For this review, use the dimensioned drawing (mm, ordinates from the lowest corner) and the shaded views. A direction names the side the tool comes from. Coordinates: 2 decimals unless noted, no trailing zeros. Order: outer loops, then holes, each group sorted by start corner. A loop starts at its lowest first (then second) coordinate and runs counter-clockwise, first axis right, second up. Notation, with made-up numbers: (67.5, -33.75) -> (122.5, -33.75) arc R36 cw to (122.5, 1.25) -> close; hole circle Ø10 at (-10, 76). An arc over 180 degrees is marked (long way). Use one line per item in the form item = value. Start each with the question number.
(1) Mouldability with a two-part tool opening along X and no side actions: class the marked faces 3, 4 and 5 as +X half, -X half, draft (parallel to the pull), parting line (faces both ways), or undercut.
(2) Take a section at C-C (y = 19). State the section outline as (x, z) points.
(3) Take a section at D-D (y = 8). State the section outline as (x, z) points, then the cut area to 3 significant figures.
(4) Take a section at A-A (x = 17.5). State the section outline as (y, z) points, then the cut area to 3 significant figures.
(5) Take a section at B-B (z = 17.5). State the section outline as (x, y) points.
(6) Wall thickness on line 1 along X through (y, z) = (20.5, 17.5); line 2 along Z through (x, y) = (17.5, 10.5): over which ranges is each line inside the solid? List them lowest first.
(7) Insertion check: pin 1 Ø4 at (y, z) = (22.5, 20) entering from +X; pin 2 Ø2 at (x, y) = (17.5, 15) entering from +Z; pin 3 Ø5 at (y, z) = (13.5, 7.5) entering from +X. Each pin has a flat end and moves straight along its axis. Give the tip position at first contact, or say it passes through.
(8) For the marked faces 1 and 2, list the 3-axis set-ups (+Z, -Z, +X, -X, +Y, -Y) from which the entire face can be reached by the end or side of a thin tool; tool diameter is ignored.
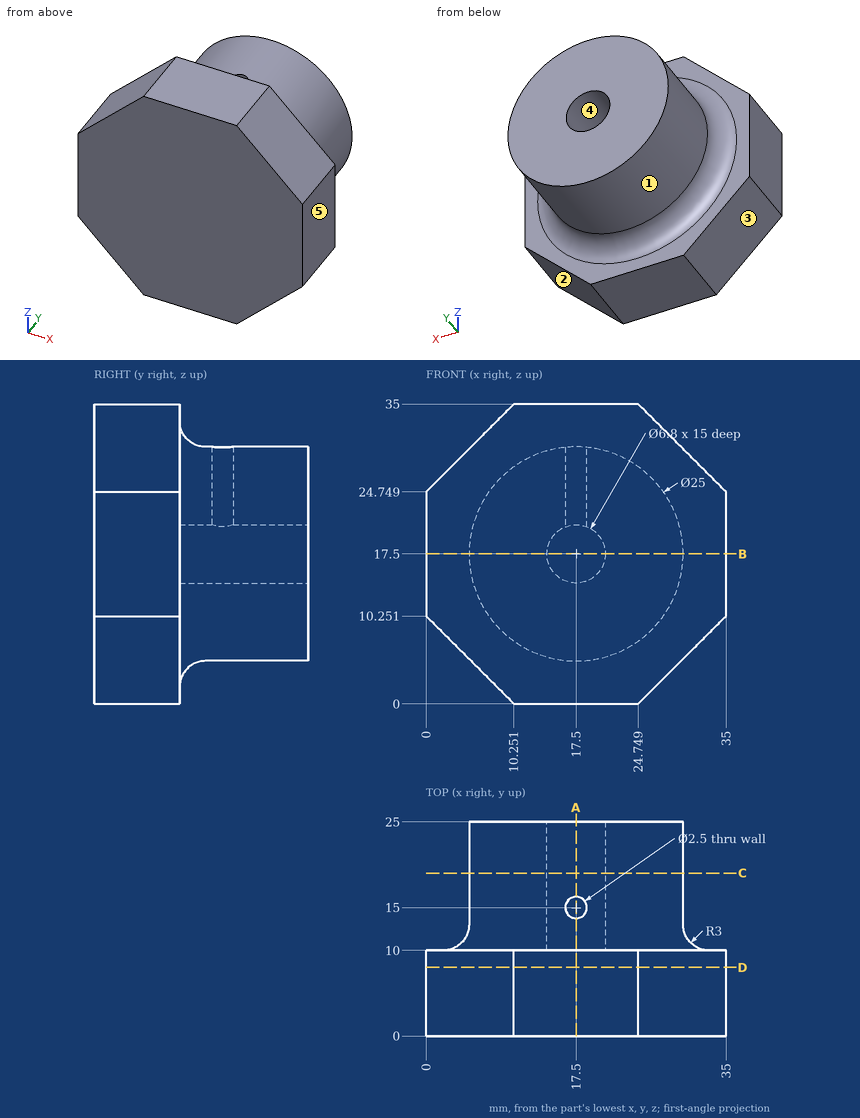
Findings:
q1.face_3 = -X half
q1.face_4 = undercut
q1.face_5 = +X half
q2.outline = circle Ø25 at (17.5, 17.5); hole circle Ø6.8 at (17.5, 17.5)
q3.outline = (0, 10.25) -> (10.25, 0) -> (24.75, 0) -> (35, 10.25) -> (35, 24.75) -> (24.75, 35) -> (10.25, 35) -> (0, 24.75) -> close
q3.area = 1,010 mm²
q4.outline = (0, 0) -> (10, 0) -> (10, 2) arc R3 cw to (13, 5) -> (25, 5) -> (25, 14.1) -> (10, 14.1) -> (10, 20.9) -> (13.75, 20.9) -> (13.75, 30) -> (13, 30) arc R3 cw to (10, 33) -> (10, 35) -> (0, 35) -> close; (16.25, 20.9) -> (25, 20.9) -> (25, 30) -> (16.25, 30) -> close
q4.area = 604 mm²
q5.outline = (0, 0) -> (35, 0) -> (35, 10) -> (33, 10) arc R3 cw to (30, 13) -> (30, 25) -> (20.9, 25) -> (20.9, 10) -> (14.1, 10) -> (14.1, 25) -> (5, 25) -> (5, 13) arc R3 cw to (2, 10) -> (0, 10) -> close
q6.line_1 = 5 to 14.1, 20.9 to 30
q6.line_2 = 3.66 to 14.1, 20.9 to 31.34
q7.pin_1 = 29.99
q7.pin_2 = 14.25
q7.pin_3 = 27.5
q8.face_1 = +Y
q8.face_2 = -Z, +X, +Y, -Y
